from build123d import *

# Parameters (mm, degrees)
BOSS_EXTRUDE1_DEPTH     = 2.5
SKETCH2_R               = 1.2
CUT_EXTRUDE1_DEPTH      = 21.676073128
SKETCH3_W               = 5
SKETCH3_H               = 15
SKETCH3_R               = 1.2
BOSS_EXTRUDE2_DEPTH     = 1.5
CUT_EXTRUDE2_REACH      = 23.852
CUT_EXTRUDE2_END_RADIUS = 6.5
CUT_EXTRUDE4_START      = -2.5
CUT_EXTRUDE4_DEPTH      = 5


# Read off the part's stored shape, not the designer's step: Cut-Extrude4
with BuildPart() as part:
    # Sketch1 → Boss-Extrude1 (new, symmetric)
    with BuildSketch(Plane.XY):
        with BuildLine():
            Line((5, 0), (11.5, 0))
            Line((11.5, 0), (11.5, -1.5))
            Line((11.5, -1.5), (6.32455532, -1.5))
            ThreePointArc((6.32455532, -1.5), (5.81561728, -2.903204376), (5, -4.153311931))
            Line((5, -4.153311931), (5, -17))
            Line((5, -17), (-5, -17))
            Line((-5, -17), (-5, -4.153311931))
            ThreePointArc((-5, -4.153311931), (-5.81561728, -2.903204376), (-6.32455532, -1.5))
            Line((-6.32455532, -1.5), (-11.5, -1.5))
            Line((-11.5, -1.5), (-11.5, 0))
            Line((-11.5, 0), (-5, 0))
            ThreePointArc((-5, 0), (0, -5), (5, 0))
        make_face()
    extrude(amount=BOSS_EXTRUDE1_DEPTH, both=True)

    # Sketch2 → Cut-Extrude1 (cut, through all)
    with BuildSketch(Plane(origin=(0, 0, 0), x_dir=(1, 0, 0), z_dir=(0, 1, 0))):
        with Locations(Location((-9, 0, 0), (0, 0, 270))):
            Circle(SKETCH2_R)
        with Locations(Location((9, 0, 0), (0, 0, 180))):
            Circle(SKETCH2_R)
    extrude(amount=-CUT_EXTRUDE1_DEPTH, mode=Mode.SUBTRACT)

    # Sketch3 → Boss-Extrude2 (add)
    with BuildSketch(Plane.XZ.offset(17)):
        Rectangle(SKETCH3_W, SKETCH3_H)
        with Locations((0, 5)):
            Circle(SKETCH3_R, mode=Mode.SUBTRACT)
        with Locations(Location((0, -5, 0), (0, 0, 180))):
            Circle(SKETCH3_R, mode=Mode.SUBTRACT)
    extrude(amount=-BOSS_EXTRUDE2_DEPTH)

    # Cut-Extrude2: up to this cylinder (the profile starts outside it)
    cut_extrude2_end = Plane(origin=(0, 0, 1.666667), z_dir=(0, 0, -1)) * Cylinder(CUT_EXTRUDE2_END_RADIUS, 61.704, mode=Mode.PRIVATE)
    # Sketch4 → Cut-Extrude2 (cut, up to the surface)
    with BuildSketch(Plane.XZ.offset(17), mode=Mode.PRIVATE) as cut_extrude2_sk1:
        Polygon((2.5, 2.5), (5, 0), (5, 2.5), align=None)
    cut_extrude2_tool1 = extrude(cut_extrude2_sk1.sketch, amount=-CUT_EXTRUDE2_REACH, mode=Mode.PRIVATE) - cut_extrude2_end
    add(cut_extrude2_tool1.solids().sort_by_distance((4.166667, -17, 1.666667))[0], mode=Mode.SUBTRACT)
    # Sketch4 → Cut-Extrude2 (cut, up to the surface)
    with BuildSketch(Plane.XZ.offset(17), mode=Mode.PRIVATE) as cut_extrude2_sk2:
        Polygon((-5, 2.5), (-2.5, 2.5), (-5, 0), align=None)
    cut_extrude2_tool2 = extrude(cut_extrude2_sk2.sketch, amount=-CUT_EXTRUDE2_REACH, mode=Mode.PRIVATE) - cut_extrude2_end
    add(cut_extrude2_tool2.solids().sort_by_distance((-4.166667, -17, 1.666667))[0], mode=Mode.SUBTRACT)

    # Cut-Extrude4 outline → Cut-Extrude4 (cut)
    with BuildSketch(Plane.XY.offset(CUT_EXTRUDE4_START)):
        with BuildLine():
            Line((-2.5, -14), (-2.5, -6))
            ThreePointArc((-2.5, -6), (-3.862002616, -5.228282299), (-5, -4.153311931))
            Line((-5, -4.153311931), (-5, -14))
            Line((-5, -14), (-2.5, -14))
        make_face()
        with BuildLine():
            Line((5, -14), (5, -4.153311931))
            ThreePointArc((5, -4.153311931), (3.862002616, -5.228282299), (2.5, -6))
            Line((2.5, -6), (2.5, -14))
            Line((2.5, -14), (5, -14))
        make_face()
    extrude(amount=CUT_EXTRUDE4_DEPTH, mode=Mode.SUBTRACT)


solid = part.part
Geometry check sheet. Reference: the model listing, model coordinates, mm. A direction names the side the tool comes from. Coordinates: 2 decimals unless noted, no trailing zeros. Order: outer loops, then holes, each group sorted by start corner. A loop starts at its lowest first (then second) coordinate and runs counter-clockwise, first axis right, second up. Notation, with made-up numbers: (87.5, 16) - (144.5, 16) arc R18 ccw to (144.5, 49) - close; hole circle Ø2 at (24.5, 25). An arc over 180 degrees is marked (long way). One line per item, written item: value.
(1) Sectioned sample at D-D (z = -3.5). Enter the section's corners in (x, y), and give its area (3 significant figures).
Data:
outline: (-2.5, -17) - (2.5, -17) - (2.5, -15.5) - (-2.5, -15.5) - close
area: 7.50 mm^2
(2) Sectioned sample at C-C (y = -3.5). Enter the section's corners in (x, z).
Data:
outline: (-5.48, -2.5) - (-3.57, -2.5) - (-3.57, 2.5) - (-5.48, 2.5) - close; (3.57, -2.5) - (5.48, -2.5) - (5.48, 2.5) - (3.57, 2.5) - close
(3) Sectioned sample at B-B (y = -16). Enter the section's corners in (x, z), and give its area (3 significant figures).
Data:
outline: (-5, -2.5) - (-2.5, -2.5) - (-2.5, -7.5) - (2.5, -7.5) - (2.5, -2.5) - (5, -2.5) - (5, 0) - (2.5, 2.5) - (2.5, 7.5) - (-2.5, 7.5) - (-2.5, 2.5) - (-5, 0) - close; hole circle Ø2.4 at (0, -5); hole circle Ø2.4 at (0, 5)
area: 84.7 mm^2
(4) Thickness scan on probe 1 along Z at (x, y) = (0, -16.4); probe 2 along Y at (x, z) = (7.75, 0); probe 3 along Z at (x, y) = (9, -0.7). Record the ranges inside material, lowest first. Write a range as from..to.
Data:
probe 1: z = -7.5..-6.2, -3.8..3.8, 6.2..7.5
probe 2: y = -1.5..0
probe 3: z = -2.5..-1.2, 1.2..2.5
(5) Sectioned sample at A-A (x = 9). Enter the section's corners in (y, z).
Data:
outline: (-1.5, -2.5) - (0, -2.5) - (0, -1.2) - (-1.5, -1.2) - close; (-1.5, 1.2) - (0, 1.2) - (0, 2.5) - (-1.5, 2.5) - close
(6) Access from +Z, -Z, +X, -X, +Y, -Y to the whole of each face (thin tool, end or side, straight path). Record for faces 1 (the face through (-2.5, -10, 0)), 2 (the face through (-5, -16, -1)), 3 (the face through (-2.5, -16, 5)), 4 (the face through (2.5, -16, 5)).
Data:
face 1: +Z, -Z, -X
face 2: +Z, -Z, -X, -Y
face 3: +Z, -X, +Y, -Y
face 4: +Z, +X, +Y, -Y
(7) Depth check by flat-ended pin: pin 1 Ø1.5 at (x, y) = (3, -8.5) entering from +Z; pin 2 Ø2 at (x, z) = (9, 0) entering from +Y; pin 3 Ø1.2 at (y, z) = (-16, 5) entering from -X; pin 4 Ø1.5 at (x, z) = (10, 1) entering from -Y. Enter the tip coordinate at first touch or a pass-through.
Data:
pin 1: stops at z = 2.5
pin 2: passes through
pin 3: stops at x = -2.5
pin 4: stops at y = -1.5
(8) Release check for a two-part mould opening along Z. For faces 5 (the face through (0, -16, -7.5)), 6 (the face through (0, -16, 7.5)), 7 (the face through (-7.6, 0, 0)), 8 (the face through (-10.17, -0.74, -0.26)) record: +Z half, -Z half, draft (parallel to the pull), parting line (faces both ways), or undercut.
Data:
face 5: -Z half
face 6: +Z half
face 7: draft
face 8: undercut
